Here's how the part is built. I have some questions about the finished solid (model axes, mm). Face numbers are marked on the shaded views. A direction names the side the tool comes from. Round coordinates to 2 decimals unless told otherwise and drop trailing zeros. Order: outer loops, then holes, each group sorted by start corner. A loop starts at its lowest first (then second) coordinate and runs counter-clockwise, first axis right, second up. Notation, with made-up numbers: (88.25, 39) -> (111.25, 39) arc R13 cw to (111.25, 55) -> close; hole circle Ø3 at (33.5, 2). An arc over 180 degrees is marked (long way). Answer in a Markdown table with one row per item.
```python
from build123d import *

# Parameters (mm, degrees)
BOSS_EXTRUDE5_DEPTH     = 18
BOSS_EXTRUDE6_START     = 17
BOSS_EXTRUDE6_DEPTH     = 1
BOSS_EXTRUDE7_START     = 5.8
SKETCH2_5_R             = 1.5
BOSS_EXTRUDE7_DEPTH     = 4
CUT_EXTRUDE1_DEPTH      = 167.833614155
CUT_EXTRUDE1_DEPTH_BACK = 167.833614155
BOSS_EXTRUDE9_START     = -1
SKETCH6_R               = 3.5
SKETCH6_R_2             = 2.25
BOSS_EXTRUDE9_DEPTH     = 6
SKETCH8_R               = 5
SKETCH8_W               = 32
SKETCH8_H               = 13
SKETCH8_W_2             = 16
SKETCH8_H_2             = 7
SKETCH8_W_3             = 10
SKETCH8_H_3             = 12
CUT_EXTRUDE2_DEPTH      = 218.268839312
CUT_EXTRUDE2_DEPTH_BACK = 6
SKETCH7_R               = 1.2
SKETCH7_R_2             = 3
SKETCH7_R_3             = 2
BOSS_EXTRUDE10_DEPTH    = 15


with BuildPart() as part:
    # Sketch2 → Boss-Extrude5 (new body)
    with BuildSketch(Plane(origin=(0, 0, 0), x_dir=(1, 0, 0), z_dir=(0, 1, 0))):
        Polygon((-76.553603822, 35.6), (-97.153603822, 35.6), (-97.153603822, 126.6), (-76.553603822, 126.6), (-76.553603822, 115.6), (30, 115.6), (30, 93), (68.5, 93), (68.5, -51.5), (26, -51.5), (26, -2), (-2, -2), (-2, 88.898979486), (-76.553603822, 88.898979486), align=None)
        Polygon((-77.553603822, 89.898979486), (-77.553603822, 36.6), (-96.157091143, 36.6), (-96.157091143, 125.6), (-77.553603822, 125.6), (-77.553603822, 114.6), (29, 114.6), (29, 92), (67.5, 92), (67.5, -50.5), (27, -50.5), (27, -1), (-1, -1), (-1, 89.898979486), align=None, mode=Mode.SUBTRACT)
    extrude(amount=BOSS_EXTRUDE5_DEPTH)

    # Sketch2<4> → Boss-Extrude6 (add)
    with BuildSketch(Plane(origin=(0, 0, 0), x_dir=(1, 0, 0), z_dir=(0, 1, 0)).offset(BOSS_EXTRUDE6_START)):
        Polygon((-77.553603822, 36.6), (-96.157091143, 36.6), (-96.157091143, 125.6), (-77.553603822, 125.6), (-77.553603822, 114.6), (29, 114.6), (29, 92), (67.5, 92), (67.5, -50.5), (27, -50.5), (27, -1), (-1, -1), (-1, 89.898979486), (-77.553603822, 89.898979486), align=None)
    extrude(amount=BOSS_EXTRUDE6_DEPTH)

    # Sketch2<5> → Boss-Extrude7 (add)
    with BuildSketch(Plane(origin=(0, 0, 0), x_dir=(1, 0, 0), z_dir=(0, 1, 0)).offset(BOSS_EXTRUDE7_START)):
        with BuildLine():
            Line((-102.153603822, 39.6), (-97.153603822, 39.6))
            Line((-97.153603822, 39.6), (-97.153603822, 49.6))
            Line((-97.153603822, 49.6), (-102.153603822, 49.6))
            ThreePointArc((-102.153603822, 49.6), (-107.153603822, 44.6), (-102.153603822, 39.6))
        make_face()
        with Locations(Location((-102.153603822, 44.6, 0), (0, 0, 270))):
            Circle(SKETCH2_5_R, mode=Mode.SUBTRACT)
        with BuildLine():
            Line((-76.553603822, 49.6), (-76.553603822, 39.6))
            Line((-76.553603822, 39.6), (-71.553603822, 39.6))
            ThreePointArc((-71.553603822, 39.6), (-66.553603822, 44.6), (-71.553603822, 49.6))
            Line((-71.553603822, 49.6), (-76.553603822, 49.6))
        make_face()
        with Locations(Location((-71.553603822, 44.6, 0), (0, 0, 270))):
            Circle(SKETCH2_5_R, mode=Mode.SUBTRACT)
        with BuildLine():
            Line((-76.553603822, 88.898979486), (-76.553603822, 79.101020514))
            Line((-76.553603822, 79.101020514), (-71.755562411, 79.004080392))
            Line((-71.755562411, 79.004080392), (-71.553603822, 79))
            ThreePointArc((-71.553603822, 79), (-68.018069917, 80.464466094), (-66.553603822, 84))
            Line((-66.553603822, 84), (-66.553603822, 88.898979486))
            Line((-66.553603822, 88.898979486), (-76.553603822, 88.898979486))
        make_face()
        with Locations(Location((-71.553603822, 84, 0), (0, 0, 270))):
            Circle(SKETCH2_5_R, mode=Mode.SUBTRACT)
        with BuildLine():
            Line((-2, 88.898979486), (-12, 88.898979486))
            Line((-12, 88.898979486), (-12, 84))
            ThreePointArc((-12, 84), (-10.535533906, 80.464466094), (-7, 79))
            Line((-7, 79), (-2, 79))
            Line((-2, 79), (-2, 88.898979486))
        make_face()
        with Locations(Location((-7, 84, 0), (0, 0, 270))):
            Circle(SKETCH2_5_R, mode=Mode.SUBTRACT)
        with BuildLine():
            Line((26, -2), (16, -2))
            Line((16, -2), (16, -7))
            ThreePointArc((16, -7), (17.464466094, -10.535533906), (21, -12))
            Line((21, -12), (26, -12))
            Line((26, -12), (26, -2))
        make_face()
        with Locations(Location((21, -7, 0), (0, 0, 270))):
            Circle(SKETCH2_5_R, mode=Mode.SUBTRACT)
        with BuildLine():
            Line((26, -49.5), (26, -39.5))
            Line((26, -39.5), (21, -39.5))
            ThreePointArc((21, -39.5), (16, -44.5), (21, -49.5))
            Line((21, -49.5), (26, -49.5))
        make_face()
        with Locations(Location((21, -44.5, 0), (0, 0, 270))):
            Circle(SKETCH2_5_R, mode=Mode.SUBTRACT)
        with BuildLine():
            Line((73.5, -39.5), (68.5, -39.5))
            Line((68.5, -39.5), (68.5, -49.5))
            Line((68.5, -49.5), (73.5, -49.5))
            ThreePointArc((73.5, -49.5), (78.5, -44.5), (73.5, -39.5))
        make_face()
        with Locations(Location((73.5, -44.5, 0), (0, 0, 270))):
            Circle(SKETCH2_5_R, mode=Mode.SUBTRACT)
        with BuildLine():
            Line((35, 103), (30, 103))
            Line((30, 103), (30, 93))
            Line((30, 93), (40, 93))
            Line((40, 93), (40, 98))
            ThreePointArc((40, 98), (38.535533906, 101.535533906), (35, 103))
        make_face()
        with Locations(Location((35, 98, 0), (0, 0, 270))):
            Circle(SKETCH2_5_R, mode=Mode.SUBTRACT)
        with BuildLine():
            Line((-102.153603822, 115.6), (-97.153603822, 115.6))
            Line((-97.153603822, 115.6), (-97.153603822, 125.6))
            Line((-97.153603822, 125.6), (-102.153603822, 125.6))
            ThreePointArc((-102.153603822, 125.6), (-107.153603822, 120.6), (-102.153603822, 115.6))
        make_face()
        with Locations(Location((-102.153603822, 120.6, 0), (0, 0, 270))):
            Circle(SKETCH2_5_R, mode=Mode.SUBTRACT)
        with BuildLine():
            Line((-71.553603822, 125.6), (-76.553603822, 125.6))
            Line((-76.553603822, 125.6), (-76.553603822, 115.6))
            Line((-76.553603822, 115.6), (-66.553603822, 115.6))
            Line((-66.553603822, 115.6), (-66.553603822, 120.6))
            ThreePointArc((-66.553603822, 120.6), (-68.018069917, 124.135533906), (-71.553603822, 125.6))
        make_face()
        with Locations(Location((-71.553603822, 120.6, 0), (0, 0, 270))):
            Circle(SKETCH2_5_R, mode=Mode.SUBTRACT)
        with Locations((73.5, 84)):
            Circle(SKETCH2_5_R)
    extrude(amount=BOSS_EXTRUDE7_DEPTH)


with BuildPart() as boss_extrude7_kept_piece:
    # of the separate pieces the step leaves, the one the design keeps (boss_extrude7_pieces_kept)
    add(part.part.solids().sort_by_distance((-76.553603822, 0, -35.6))[0])

    # Sketch5 → Cut-Extrude1 (cut, two sides)
    with BuildSketch(Plane(origin=(0, 18, 0), x_dir=(1, 0, 0), z_dir=(0, 1, 0))) as cut_extrude1_sk:
        with BuildLine():
            Line((-86.781104823, 121.7), (-84.514671921, 121.7))
            Line((-84.514671921, 121.7), (-84.514671921, 120.7))
            Line((-84.514671921, 120.7), (-87.305527611, 120.7))
            ThreePointArc((-87.305527611, 120.7), (-92.903603822, 119.2), (-87.305527611, 117.7))
            Line((-87.305527611, 117.7), (-84.514671921, 117.7))
            Line((-84.514671921, 117.7), (-84.514671921, 116.7))
            Line((-84.514671921, 116.7), (-86.781104823, 116.7))
            ThreePointArc((-86.781104823, 116.7), (-93.903603822, 119.2), (-86.781104823, 121.7))
        make_face()
        with BuildLine():
            Line((-86.781104823, 103.35), (-84.514671921, 103.35))
            Line((-84.514671921, 103.35), (-84.514671921, 102.35))
            Line((-84.514671921, 102.35), (-87.305527611, 102.35))
            ThreePointArc((-87.305527611, 102.35), (-92.903603822, 100.85), (-87.305527611, 99.35))
            Line((-87.305527611, 99.35), (-84.514671921, 99.35))
            Line((-84.514671921, 99.35), (-84.514671921, 98.35))
            Line((-84.514671921, 98.35), (-86.781104823, 98.35))
            ThreePointArc((-86.781104823, 98.35), (-93.903603822, 100.85), (-86.781104823, 103.35))
        make_face()
        with BuildLine():
            Line((-86.781104823, 91.35), (-84.514671921, 91.35))
            Line((-84.514671921, 91.35), (-84.514671921, 90.35))
            Line((-84.514671921, 90.35), (-87.305527611, 90.35))
            ThreePointArc((-87.305527611, 90.35), (-92.903603822, 88.85), (-87.305527611, 87.35))
            Line((-87.305527611, 87.35), (-84.514671921, 87.35))
            Line((-84.514671921, 87.35), (-84.514671921, 86.35))
            Line((-84.514671921, 86.35), (-86.781104823, 86.35))
            ThreePointArc((-86.781104823, 86.35), (-93.903603822, 88.85), (-86.781104823, 91.35))
        make_face()
        with BuildLine():
            Line((-86.781104823, 76), (-84.514671921, 76))
            Line((-84.514671921, 76), (-84.514671921, 75))
            Line((-84.514671921, 75), (-87.305527611, 75))
            ThreePointArc((-87.305527611, 75), (-92.903603822, 73.5), (-87.305527611, 72))
            Line((-87.305527611, 72), (-84.514671921, 72))
            Line((-84.514671921, 72), (-84.514671921, 71))
            Line((-84.514671921, 71), (-86.781104823, 71))
            ThreePointArc((-86.781104823, 71), (-93.903603822, 73.5), (-86.781104823, 76))
        make_face()
        with BuildLine():
            Line((-86.781104823, 56.5), (-84.514671921, 56.5))
            Line((-84.514671921, 56.5), (-84.514671921, 55.5))
            Line((-84.514671921, 55.5), (-87.305527611, 55.5))
            ThreePointArc((-87.305527611, 55.5), (-92.903603822, 54), (-87.305527611, 52.5))
            Line((-87.305527611, 52.5), (-84.514671921, 52.5))
            Line((-84.514671921, 52.5), (-84.514671921, 51.5))
            Line((-84.514671921, 51.5), (-86.781104823, 51.5))
            ThreePointArc((-86.781104823, 51.5), (-93.903603822, 54), (-86.781104823, 56.5))
        make_face()
    extrude(amount=CUT_EXTRUDE1_DEPTH, mode=Mode.SUBTRACT)
    extrude(cut_extrude1_sk.sketch, amount=-CUT_EXTRUDE1_DEPTH_BACK, mode=Mode.SUBTRACT)

    # Sketch6 → Boss-Extrude9 (add)
    with BuildSketch(Plane(origin=(0, 18, 0), x_dir=(1, 0, 0), z_dir=(0, 1, 0)).offset(BOSS_EXTRUDE9_START)):
        with Locations(Location((-89.903603822, 109.25, 0), (0, 0, 270))):
            Circle(SKETCH6_R)
        with Locations(Location((-89.903603822, 109.25, 0), (0, 0, 270))):
            Circle(SKETCH6_R_2, mode=Mode.SUBTRACT)
        with Locations(Location((-89.903603822, 63, 0), (0, 0, 270))):
            Circle(SKETCH6_R)
        with Locations(Location((-89.903603822, 63, 0), (0, 0, 270))):
            Circle(SKETCH6_R_2, mode=Mode.SUBTRACT)
    extrude(amount=-BOSS_EXTRUDE9_DEPTH)

    # Sketch8 → Cut-Extrude2 (cut, two sides)
    with BuildSketch(Plane(origin=(68.5, 0, 0), x_dir=(0, 0, -1), z_dir=(1, 0, 0))) as cut_extrude2_sk:
        with Locations((80.5, 9.4)):
            Circle(SKETCH8_R)
        with Locations((58, 8.5)):
            Rectangle(SKETCH8_W, SKETCH8_H)
        with Locations((31, 5.5)):
            Rectangle(SKETCH8_W_2, SKETCH8_H_2)
        with Locations((9, 8)):
            Rectangle(SKETCH8_W_3, SKETCH8_H_3)
    extrude(amount=CUT_EXTRUDE2_DEPTH, mode=Mode.SUBTRACT)
    extrude(cut_extrude2_sk.sketch, amount=-CUT_EXTRUDE2_DEPTH_BACK, mode=Mode.SUBTRACT)

    # Sketch7 → Boss-Extrude10 (add)
    with BuildSketch(Plane.XZ.offset(-17)):
        with Locations(Location((1.2, -10.7, 0), (0, 0, 90))):
            Circle(SKETCH7_R)
        with Locations(Location((2, -89, 0), (0, 0, 90))):
            Circle(SKETCH7_R)
        with Locations(Location((63.3, -88.4, 0), (0, 0, 90))):
            Circle(SKETCH7_R)
        with Locations(Location((63, -1.6, 0), (0, 0, 90))):
            Circle(SKETCH7_R)
        with Locations(Location((52.066768514, -32.967079536, 0), (0, 0, 90))):
            Circle(SKETCH7_R_2)
        with Locations(Location((3, -52, 0), (0, 0, 90))):
            Circle(SKETCH7_R_3)
    extrude(amount=BOSS_EXTRUDE10_DEPTH)


solid = boss_extrude7_kept_piece.part
```
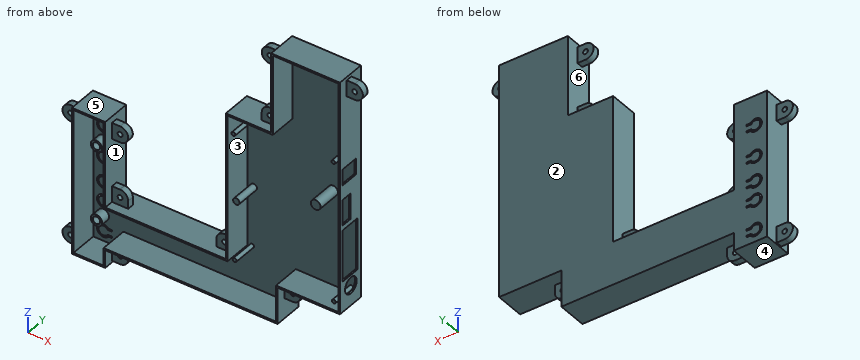
1. For the marked faces 1, 2 and 3, which set-ups out of +Z, -Z, +X, -X, +Y, -Y let a thin tool reach every point of the face, with its end or its side?
Numbers:
| item | result |
|---|---|
| face 1 | none |
| face 2 | +Z, -Z, +X, -X, +Y |
| face 3 | -Y |
2. For pin 1 Ø2 at (x, y) = (-31.5, 5) entering from -Z; pin 2 Ø0.5 at (x, y) = (-85.5, 17.5) entering from +Z; pin 3 Ø1 at (y, z) = (9, -97.5) entering from -X; pin 4 Ø3.5 at (y, z) = (8.5, -121.5) entering from -X, each with a flat end and sliding along its axis, tell me the tip position at first contact or that it passes through.
Numbers:
| item | result |
|---|---|
| pin 1 | stops at z = -115.6 |
| pin 2 | stops at z = -35.6 |
| pin 3 | stops at x = -97.15 |
| pin 4 | stops at x = -107.15 |
3. We'd pull the mould along Z, two halves only. Please class the marked faces 4, 5 and 6: released by +Z, released by -Z, zero draft, split by the parting line, or undercut.
Numbers:
| item | result |
|---|---|
| face 4 | released by -Z |
| face 5 | released by +Z |
| face 6 | undercut |
4. Please list where these lines run through material, in increasing order: line 1 along X through (y, z) = (14.5, -39); line 2 along X through (y, z) = (7.1, 7); line 3 along X through (y, z) = (7.85, -98).
Numbers:
| item | result |
|---|---|
| line 1 | x = -97.15 to -96.16, -77.55 to -76.55, -2 to -1, 67.5 to 68.5 |
| line 2 | x = 16 to 19.5, 22.5 to 27, 67.5 to 68.5 |
| line 3 | x = -97.15 to -96.16, 29 to 33.5, 36.5 to 40 |
5. Suppose I cut it at A-A on z = 23.5. Write out the boundary of the cut face in (x, y), then the cut area to 3 significant figures.
Numbers:
| item | result |
|---|---|
| outline | (26, 0) -> (27, 0) -> (27, 17) -> (67.5, 17) -> (67.5, 0) -> (68.5, 0) -> (68.5, 18) -> (26, 18) -> close |
| area | 76.5 mm2 |
